The listing builds one solid part. Answer for the finished solid, in the listing's coordinates (mm). A direction names the side the tool comes from. Give positions to 0.01 mm unless a question says otherwise; leave off trailing zeros. Order: outer loops, then holes, each group sorted by start corner. A loop starts at its lowest first (then second) coordinate and runs counter-clockwise, first axis right, second up. Notation, with made-up numbers: (72, 3.5) - (128, 3.5) arc R9 ccw to (128, 17.5) - close; hole circle Ø1 at (74, 62.5). An arc over 180 degrees is marked (long way). Use CSV: the item, a comma, the result in double quotes.
```python
from build123d import *

# Parameters (mm, degrees)
SKETCH1_W           = 98
SKETCH1_H           = 98
BOSS_EXTRUDE2_DEPTH = 5
SKETCH12_W          = 88
SKETCH12_H          = 88
SKETCH12_W_2        = 78
SKETCH12_H_2        = 78
BOSS_EXTRUDE4_DEPTH = 2
SKETCH13_R          = 1.75
CUT_EXTRUDE13_DEPTH = 2
SKETCH14_R          = 1
CUT_EXTRUDE14_DEPTH = 9
SKETCH16_W          = 62
SKETCH16_H          = 62
CUT_EXTRUDE15_DEPTH = 3
FILLET1_R           = 3
SKETCH17_R          = 1.5
CUT_EXTRUDE16_DEPTH = 3
SKETCH23_W          = 6
SKETCH23_H          = 15
CUT_EXTRUDE19_DEPTH = 12
FILLET2_R           = 1
SKETCH24_R          = 2
CUT_EXTRUDE22_DEPTH = 12


with BuildPart() as part:
    # Sketch1 → Boss-Extrude2 (new body)
    with BuildSketch(Plane(origin=(0, 0, 0), x_dir=(1, 0, 0), z_dir=(0, 1, 0))):
        Rectangle(SKETCH1_W, SKETCH1_H)
    extrude(amount=BOSS_EXTRUDE2_DEPTH)

    # Sketch12 → Boss-Extrude4 (add)
    with BuildSketch(Plane.XZ):
        Rectangle(SKETCH12_W, SKETCH12_H)
        Rectangle(SKETCH12_W_2, SKETCH12_H_2, mode=Mode.SUBTRACT)
    extrude(amount=BOSS_EXTRUDE4_DEPTH)

    # Sketch13 → Cut-Extrude13 (cut)
    with BuildSketch(Plane(origin=(0, 5, 0), x_dir=(1, 0, 0), z_dir=(0, 1, 0))):
        with BuildLine():
            ThreePointArc((0, -44.75), (-1.75, -46.5), (0, -48.25))
            Line((0, -48.25), (0, -44.75))
        make_face()
        with BuildLine():
            Line((0, -44.75), (0, -48.25))
            ThreePointArc((0, -48.25), (1.237436867, -47.737436867), (1.75, -46.5))
            ThreePointArc((1.75, -46.5), (1.237436867, -45.262563133), (0, -44.75))
        make_face()
        with Locations(Location((-46.5, 0, 0), (0, 0, 270))):
            Circle(SKETCH13_R)
        with Locations(Location((0, 46.5, 0), (0, 0, 270))):
            Circle(SKETCH13_R)
        with BuildLine():
            ThreePointArc((44.75, 0), (46.5, -1.75), (48.25, 0))
            Line((48.25, 0), (44.75, 0))
        make_face()
        with BuildLine():
            Line((44.75, 0), (48.25, 0))
            ThreePointArc((48.25, 0), (46.5, 1.75), (44.75, 0))
        make_face()
    extrude(amount=-CUT_EXTRUDE13_DEPTH, mode=Mode.SUBTRACT)

    # Sketch14 → Cut-Extrude14 (cut)
    with BuildSketch(Plane(origin=(0, 5, 0), x_dir=(1, 0, 0), z_dir=(0, 1, 0))):
        with Locations(Location((0, -46.5, 0), (0, 0, 270))):
            Circle(SKETCH14_R)
        with Locations(Location((-46.5, 0, 0), (0, 0, 270))):
            Circle(SKETCH14_R)
        with Locations(Location((46.5, 0, 0), (0, 0, 270))):
            Circle(SKETCH14_R)
        with Locations(Location((0, 46.5, 0), (0, 0, 270))):
            Circle(SKETCH14_R)
    extrude(amount=-CUT_EXTRUDE14_DEPTH, mode=Mode.SUBTRACT)

    # Sketch16 → Cut-Extrude15 (cut)
    with BuildSketch(Plane(origin=(0, 5, 0), x_dir=(1, 0, 0), z_dir=(0, 1, 0))):
        Rectangle(SKETCH16_W, SKETCH16_H)
    extrude(amount=-CUT_EXTRUDE15_DEPTH, mode=Mode.SUBTRACT)

    # Fillet1
    fillet1_edges = [part.edges().sort_by_distance(p)[0] for p in [
        (31, 3.5, -31),
        (31, 3.5, 31),
        (-31, 3.5, 31),
        (-31, 3.5, -31),
    ]]
    fillet(fillet1_edges, radius=FILLET1_R)

    # Sketch17 → Cut-Extrude16 (cut)
    with BuildSketch(Plane(origin=(0, 2, 0), x_dir=(1, 0, 0), z_dir=(0, 1, 0))):
        with Locations(Location((25, 25, 0), (0, 0, 270))):
            Circle(SKETCH17_R)
        with Locations(Location((25, -25, 0), (0, 0, 270))):
            Circle(SKETCH17_R)
        with Locations(Location((-25, 25, 0), (0, 0, 270))):
            Circle(SKETCH17_R)
        with Locations(Location((-25, -25, 0), (0, 0, 270))):
            Circle(SKETCH17_R)
    extrude(amount=-CUT_EXTRUDE16_DEPTH, mode=Mode.SUBTRACT)

    # Sketch23 → Cut-Extrude19 (cut)
    with BuildSketch(Plane(origin=(0, 5, 0), x_dir=(1, 0, 0), z_dir=(0, 1, 0))):
        with Locations((36, 18)):
            Rectangle(SKETCH23_W, SKETCH23_H)
        with Locations((36, 0)):
            Rectangle(SKETCH23_W, SKETCH23_H)
        with Locations((36, -18)):
            Rectangle(SKETCH23_W, SKETCH23_H)
        with Locations((-36, 18)):
            Rectangle(SKETCH23_W, SKETCH23_H)
        with Locations((-36, 0)):
            Rectangle(SKETCH23_W, SKETCH23_H)
        with Locations((-36, -18)):
            Rectangle(SKETCH23_W, SKETCH23_H)
    extrude(amount=-CUT_EXTRUDE19_DEPTH, mode=Mode.SUBTRACT)

    # Fillet2
    fillet2_edges = [part.edges().sort_by_distance(p)[0] for p in [
        (39, 2.5, 7.5),
        (33, 2.5, 7.5),
        (33, 2.5, -7.5),
        (39, 2.5, -7.5),
        (39, 2.5, 10.5),
        (39, 2.5, 25.5),
        (33, 2.5, 25.5),
        (33, 2.5, 10.5),
        (-33, 2.5, -25.5),
        (-33, 2.5, -10.5),
        (-39, 2.5, -10.5),
        (-39, 2.5, -25.5),
        (-33, 2.5, -7.5),
        (-33, 2.5, 7.5),
        (-39, 2.5, 7.5),
        (-39, 2.5, -7.5),
        (-39, 2.5, 10.5),
        (-33, 2.5, 10.5),
        (-33, 2.5, 25.5),
        (-39, 2.5, 25.5),
        (39, 2.5, -25.5),
        (39, 2.5, -10.5),
        (33, 2.5, -10.5),
        (33, 2.5, -25.5),
    ]]
    fillet(fillet2_edges, radius=FILLET2_R)

    # Sketch24 → Cut-Extrude22 (cut)
    with BuildSketch(Plane(origin=(0, 5, 0), x_dir=(1, 0, 0), z_dir=(0, 1, 0))):
        with Locations(Location((0, 35, 0), (0, 0, 270))):
            Circle(SKETCH24_R)
    extrude(amount=-CUT_EXTRUDE22_DEPTH, mode=Mode.SUBTRACT)


solid = part.part
```
Item 1: The part is cut by section A-A (z = -35). Give the vertices of the cut face in (x, y).
Taken from the geometry:
outline,"(-49, 0) - (-44, 0) - (-44, -2) - (-39, -2) - (-39, 0) - (-2, 0) - (-2, 5) - (-49, 5) - close; (2, 0) - (39, 0) - (39, -2) - (44, -2) - (44, 0) - (49, 0) - (49, 5) - (2, 5) - close"
Item 2: The mould has two halves that part along Z. Classify faces 4 (the face through (-36, 3, -10.5)), 5 (the face through (-1, 2, -49)), 6 (the face through (-36, 3, 7.5)), 7 (the face through (49, 2, 1)): +Z half, -Z half, draft (parallel to the pull), parting line (faces both ways), or undercut.
Taken from the geometry:
face 4,"undercut"
face 5,"-Z half"
face 6,"undercut"
face 7,"draft"
Item 3: The part is cut by section B-B (x = 25). Give the vertices of the cut face in (y, z).
Taken from the geometry:
outline,"(-2, -44) - (0, -44) - (0, -49) - (5, -49) - (5, -31) - (2, -31) - (2, -26.5) - (0, -26.5) - (0, -39) - (-2, -39) - close; (-2, 39) - (0, 39) - (0, 26.5) - (2, 26.5) - (2, 31) - (5, 31) - (5, 49) - (0, 49) - (0, 44) - (-2, 44) - close; (0, -23.5) - (2, -23.5) - (2, 23.5) - (0, 23.5) - close"
Item 4: Which of the six approach directions +Z, -Z, +X, -X, +Y, -Y give full straight-line access (tool end or side, diameter ignored) to faces 1 (the face through (-49, 2, 1)), 2 (the face through (31, 4, 0)), 3 (the face through (36, 3, 25.5))?
Taken from the geometry:
face 1,"+Z, -Z, -X, +Y, -Y"
face 2,"+Y"
face 3,"+Y, -Y"
Item 5: Find the intervals of material crossed by line 1 along X through (y, z) = (4.4, 0); line 2 along X through (y, z) = (0.5, 22); line 3 along X through (y, z) = (1.8, 0), in increasing order.
Taken from the geometry:
line 1,"-49 to -48.25, -44.75 to -39, -33 to -31, 31 to 33, 39 to 44.75, 48.25 to 49"
line 2,"-49 to -39, -33 to 33, 39 to 49"
line 3,"-49 to -47.5, -45.5 to -39, -33 to 33, 39 to 45.5, 47.5 to 49"
Item 6: Each of these flat-tipped pins is pushed along its axis until it touches: pin 1 (1 mm diameter, centred on x = 38.5, y = -1, fed in from -Z); pin 2 (5 mm diameter, centred on x = 13, z = 11.5, fed in from -Y); pin 3 (3.5 mm diameter, centred on x = 0, z = -35, fed in from +Y); pin 4 (0.6 mm diameter, centred on y = -1, z = -16.5, fed in from +X). Where does it stop, or does it pass through?
Taken from the geometry:
pin 1,"z = -44"
pin 2,"y = 0"
pin 3,"through"
pin 4,"x = 44"
